Build history of the part. All positions in model axes, mm. Round coordinates to 2 decimals unless told otherwise and drop trailing zeros. Order: outer loops, then holes, each group sorted by start corner. A loop starts at its lowest first (then second) coordinate and runs counter-clockwise, first axis right, second up. Notation, with made-up numbers: (29.5, 39.25) -> (64.5, 39.25) arc R21 cw to (64.5, 68.25) -> close; hole circle Ø10 at (77.5, -6.75). An arc over 180 degrees is marked (long way). Write item = value, one per line.
from build123d import *

# Parameters (mm, degrees)
PAD_DEPTH                     = 8.6
PAD001_DEPTH                  = 4
SKETCH002_W                   = 1.4
SKETCH002_H                   = 94.4
POCKET001_DEPTH               = 1.5
SKETCH003_W                   = 25.4
SKETCH003_H                   = 80.4
POCKET_DEPTH                  = 8.6
SKETCH009_R                   = 3.3782
POCKET008_DEPTH               = 8.601
SKETCH008_R                   = 2.0955
POCKET005_DEPTH               = 7
SKETCH008_MIRRORED004_2_R     = 2.0955
POCKET005_MIRRORED004_2_DEPTH = 7
SKETCH010_W                   = 12
SKETCH010_H                   = 7
POCKET007_DEPTH               = 2.8


with BuildPart() as part:
    # Sketch → Pad (new body)
    with BuildSketch(Plane.XY):
        with BuildLine():
            Line((-33.1, 45.2), (-33.1, -45.2))
            ThreePointArc((-33.1, -45.2), (-32.514214, -46.614214), (-31.1, -47.2))
            Line((-31.1, -47.2), (31.1, -47.2))
            ThreePointArc((31.1, -47.2), (32.514214, -46.614214), (33.1, -45.2))
            Line((33.1, -45.2), (33.1, 45.2))
            ThreePointArc((33.1, 45.2), (32.514214, 46.614214), (31.1, 47.2))
            Line((31.1, 47.2), (-31.1, 47.2))
            ThreePointArc((-31.1, 47.2), (-32.514214, 46.614214), (-33.1, 45.2))
        make_face()
    extrude(amount=PAD_DEPTH)

    # Sketch007 → Pad001 (join)
    with BuildSketch(Plane.XY):
        with BuildLine():
            Line((-60.2375, 45.2), (-60.2375, -45.2))
            ThreePointArc((-60.2375, -45.2), (-59.651714, -46.614214), (-58.2375, -47.2))
            Line((-58.2375, -47.2), (58.2375, -47.2))
            ThreePointArc((58.2375, -47.2), (59.651714, -46.614214), (60.2375, -45.2))
            Line((60.2375, -45.2), (60.2375, 45.2))
            ThreePointArc((60.2375, 45.2), (59.651714, 46.614214), (58.2375, 47.2))
            Line((58.2375, 47.2), (-58.2375, 47.2))
            ThreePointArc((-58.2375, 47.2), (-59.651714, 46.614214), (-60.2375, 45.2))
        make_face()
    extrude(amount=PAD001_DEPTH)

    # Sketch002 (on DatumPlane) → Pocket001 (cut)
    with BuildSketch(Plane.XY.offset(8.6)):
        Rectangle(SKETCH002_W, SKETCH002_H)
    extrude(amount=-POCKET001_DEPTH, mode=Mode.SUBTRACT)

    # Sketch003 (on DatumPlane) → Pocket (cut)
    with BuildSketch(Plane.XY.offset(8.6)):
        with Locations((-13.4, 0)):
            Rectangle(SKETCH003_W, SKETCH003_H)
    pocket = extrude(amount=-POCKET_DEPTH, mode=Mode.SUBTRACT)

    # Mirrored: Pocket across Sketch003 V_Axis
    add(pocket.mirror(Plane(origin=(0, 0, 8.6), x_dir=(0, 0, 1), z_dir=(1, 0, 0))), mode=Mode.SUBTRACT)

    # Sketch009 → Pocket008 (cut, through all)
    with BuildSketch(Plane.XY):
        with Locations((-50.8, 38.1)):
            Circle(SKETCH009_R)
        with Locations((50.8, 38.1)):
            Circle(SKETCH009_R)
        with Locations((-50.8, -38.1)):
            Circle(SKETCH009_R)
        with Locations((50.8, -38.1)):
            Circle(SKETCH009_R)
    extrude(amount=POCKET008_DEPTH, mode=Mode.SUBTRACT)

    # Sketch008 (on DatumPlane) → Pocket005 (cut)
    with BuildSketch(Plane.XY.offset(8.6)):
        with Locations((-29.6, 23.6)):
            Circle(SKETCH008_R)
    pocket005 = extrude(amount=-POCKET005_DEPTH, mode=Mode.SUBTRACT)

    # Sketch008 Mirrored004 2 → Pocket005 Mirrored004 2 (cut)
    with BuildSketch(Plane(origin=(0, 0, 8.6), x_dir=(-1, 0, 0), z_dir=(0, 0, -1))):
        with Locations((-29.6, 23.6)):
            Circle(SKETCH008_MIRRORED004_2_R)
    pocket005_mirrored004_2 = extrude(amount=POCKET005_MIRRORED004_2_DEPTH, mode=Mode.SUBTRACT)

    # Mirrored005: Pocket005, Pocket005 Mirrored004 2 across XZ
    add(pocket005.mirror(Plane.XZ), mode=Mode.SUBTRACT)
    add(pocket005_mirrored004_2.mirror(Plane.XZ), mode=Mode.SUBTRACT)

    # Sketch010 → Pocket007 (cut)
    with BuildSketch(Plane.XY):
        with Locations((-13.4, 43.7)):
            Rectangle(SKETCH010_W, SKETCH010_H)
    pocket007 = extrude(amount=POCKET007_DEPTH, mode=Mode.SUBTRACT)

    # Mirrored006: Pocket007 across Sketch010 V_Axis
    add(pocket007.mirror(Plane(origin=(0, 0, 0), x_dir=(0, 0, 1), z_dir=(1, 0, 0))), mode=Mode.SUBTRACT)


solid = part.part
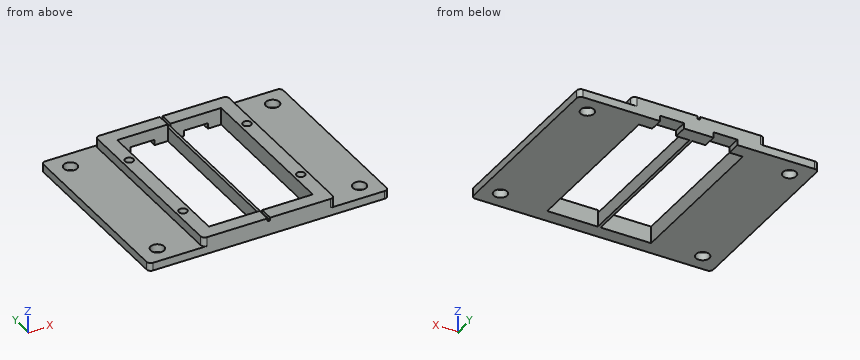
Q1. Flat gauge pins, fed straight in: pin 1 (2.5 mm diameter, centred on x = 29.6, y = 23.6, fed in from +Z); pin 2 (0.8 mm diameter, centred on y = -42, z = 8, fed in from -X); pin 3 (8.5 mm diameter, centred on x = -49.5, y = 14, fed in from +Z); pin 4 (8 mm diameter, centred on x = 43.5, y = -7.5, fed in from -Z). Where does each tip first touch, or does it go through?
Check values:
pin_1 = 1.6
pin_2 = -33.1
pin_3 = 4
pin_4 = 0
Q2. Probe probe 1 along X at (y, z) = (-35, 5); probe 2 along X at (y, z) = (-38.1, 1.2); probe 3 along Y at (x, z) = (50.8, 3.25). List the from-to ranges inside material, lowest first.
Check values:
probe_1 = -33.1 to -26.1, -0.7 to 0.7, 26.1 to 33.1
probe_2 = -60.24 to -54.18, -47.42 to -26.1, -0.7 to 0.7, 26.1 to 47.42, 54.18 to 60.24
probe_3 = -47.2 to -41.48, -34.72 to 34.72, 41.48 to 47.2
Q3. Cut at B-B, the plane x = 50.8. List the corners of the cut face in (y, z).
Check values:
outline = (-47.2, 0) -> (-41.48, 0) -> (-41.48, 4) -> (-47.2, 4) -> close; (-34.72, 0) -> (34.72, 0) -> (34.72, 4) -> (-34.72, 4) -> close; (41.48, 0) -> (47.2, 0) -> (47.2, 4) -> (41.48, 4) -> close
Q4. Cut at A-A, the plane y = 38.1. List the corners of the cut face in (x, z), and give its area (3 significant figures).
Check values:
outline = (-60.24, 0) -> (-54.18, 0) -> (-54.18, 4) -> (-60.24, 4) -> close; (-47.42, 0) -> (-26.1, 0) -> (-26.1, 8.6) -> (-33.1, 8.6) -> (-33.1, 4) -> (-47.42, 4) -> close; (-0.7, 0) -> (0.7, 0) -> (0.7, 7.1) -> (-0.7, 7.1) -> close; (26.1, 0) -> (47.42, 0) -> (47.42, 4) -> (33.1, 4) -> (33.1, 8.6) -> (26.1, 8.6) -> close; (54.18, 0) -> (60.24, 0) -> (60.24, 4) -> (54.18, 4) -> close
area = 293 mm²
Q5. Cut at D-D, the plane y = -4.5. List the corners of the cut face in (x, z), and give its area (3 significant figures).
Check values:
outline = (-60.24, 0) -> (-26.1, 0) -> (-26.1, 8.6) -> (-33.1, 8.6) -> (-33.1, 4) -> (-60.24, 4) -> close; (-0.7, 0) -> (0.7, 0) -> (0.7, 7.1) -> (-0.7, 7.1) -> close; (26.1, 0) -> (60.24, 0) -> (60.24, 4) -> (33.1, 4) -> (33.1, 8.6) -> (26.1, 8.6) -> close
area = 347 mm²
Q6. Cut at C-C, the plane z = 5.5. List the corners of the cut face in (x, y).
Check values:
outline = (-33.1, -45.2) arc R2 ccw to (-31.1, -47.2) -> (31.1, -47.2) arc R2 ccw to (33.1, -45.2) -> (33.1, 45.2) arc R2 ccw to (31.1, 47.2) -> (-31.1, 47.2) arc R2 ccw to (-33.1, 45.2) -> close; hole circle Ø4.19 at (-29.6, -23.6); hole circle Ø4.19 at (-29.6, 23.6); hole (-26.1, -40.2) -> (-0.7, -40.2) -> (-0.7, 40.2) -> (-26.1, 40.2) -> close; hole (0.7, -40.2) -> (26.1, -40.2) -> (26.1, 40.2) -> (0.7, 40.2) -> close; hole circle Ø4.19 at (29.6, -23.6); hole circle Ø4.19 at (29.6, 23.6)
